Autodesk Fusion 360 part; units mm, degrees
sketch "Sketch1" plane through (0, 0, 0) normal (0, 0, 1) x (1, 0, 0)
  line L0 (30, 50) -> (30, 22)
  line L1 (30, 22) -> (150, 22)
  line L2 (150, 22) -> (30, 50)
  dimension "d1" = 28
  dimension "d2" = 120
extrude "Extrude1" add sketch "Sketch1" along normal blind 20
sketch "Sketch2" plane through (0, 22, 0) normal (0, -1, 0) x (1, 0, 0)
  line L0 (30, 0) -> (150, 0)
  line L1 (150, 0) -> (150, 20)
  line L2 (150, 20) -> (30, 20)
  line L3 (30, 20) -> (30, 0)
  line L4 (30, 10) -> (150, 10)
  line L5 (150, 10) -> (120, 10)
  circle A0 centre (120, 10) radius 2.5
  circle A1 centre (65, 10) radius 2.5
  dimension "d5" = 30
  dimension "d6" = 5
  dimension "d7" = 5
extrude "Extrude2" cut sketch "Sketch2" against normal blind 50 contours L4 A1 | L4 A1 | L4 L5 A0 | L4 L5 A0
sketch "Sketch3" plane through (0, 0, 20) normal (0, 0, 1) x (-1, 0, 0)
  line L0 (-150, -22) -> (-30, -50)
  line L1 (-30, -50) -> (-30, -22)
  line L2 (-30, -22) -> (-150, -22)
  line L3 (-30, -50) -> (-150, -50)
  line L4 (-150, -50) -> (-150, -22)
sketch "Sketch4" plane through (0, 22, 0) normal (0, -1, 0) x (1, 0, 0)
  circle A0 centre (65, 10) radius 2.5
  circle A1 centre (120, 10) radius 2.5
  line L0 (30, 0) -> (150, 0)
  line L1 (150, 0) -> (150, 20)
  line L2 (150, 20) -> (30, 20)
  line L3 (30, 20) -> (30, 0)
  line L4 (65, 10) -> (65, 20)
  line L5 (120, 10) -> (120, 20)
sketch "Sketch5" plane through (0, 0, 20) normal (0, 0, 1) x (-1, 0, 0)
  line L0 (-120, -22) -> (-120, -50)
  line L1 (-120, -50) -> (-65, -22)
  line L2 (-65, -22) -> (-65, -50)
sketch "Sketch6" plane through (90, 22, 10) normal (0, -1, 0) x (1, 0, 0)
  line L0 (30, 14.4) -> (40.6132, 4.6089)
sketch "Sketch7" plane through (0, 0, 0) normal (0, 0, -1) x (1, 0, 0)
  line L0 (30, -50) -> (150, -22)
  line L1 (150, -22) -> (30, -22)
  line L2 (30, -22) -> (30, -50)
Geometry check sheet. Reference: the model listing, model coordinates, mm. Give positions to 0.01 mm unless a question says otherwise; leave off trailing zeros. Loops run counter-clockwise (first coordinate to the right, second up) from the corner with the lowest first, then second, coordinate; pieces in that order, holes last.
(1) Section check A-A on x = 120. Record the cut outline in (y, z), then the cut area to 3 significant figures.
From the geometry:
outline: (22, 0) - (29, 0) - (29, 7.5) - (22, 7.5) - close; (22, 12.5) - (29, 12.5) - (29, 20) - (22, 20) - close
area: 105 mm2
(2) Thickness scan on L1, parallel to Z at x = 120, y = 27.25; L2, parallel to Y at x = 87, z = 10; L3, parallel to Y at x = 129, z = 16.5. Record the ranges inside material, lowest first.
From the geometry:
L1: z = 0 to 7.5, 12.5 to 20
L2: y = 22 to 36.7
L3: y = 22 to 26.9
(3) Section check C-C on z = 10. Record the cut outline in (x, y).
From the geometry:
outline: (30, 22) - (62.5, 22) - (62.5, 42.42) - (30, 50) - close; (67.5, 22) - (117.5, 22) - (117.5, 29.58) - (67.5, 41.25) - close; (122.5, 22) - (150, 22) - (122.5, 28.42) - close
(4) Section check D-D on y = 27. Record the cut outline in (x, z).
From the geometry:
outline: (30, 0) - (128.57, 0) - (128.57, 20) - (30, 20) - close; hole circle Ø5 at (65, 10); hole circle Ø5 at (120, 10)
(5) Depth check by flat-ended pin: pin 1 Ø3 at (x, z) = (61.5, 3) entering from +Y; pin 2 Ø8 at (x, z) = (65, 10) entering from +Y. Enter the tip coordinate at first touch or a pass-through.
From the geometry:
pin 1: stops at y = 43
pin 2: stops at y = 42.77
(6) Section check B-B on y = 37.75. Record the cut outline in (x, z).
From the geometry:
outline: (30, 0) - (82.5, 0) - (82.5, 20) - (30, 20) - close; hole circle Ø5 at (65, 10)
(7) Release check for a two-part mould opening along X. For faces 1 (the flat face through (90.84, 35.804, 9.86)), 2 (the flat face through (89, 22, 10)), 3 (the cylindrical face through (118, 25.7, 8.5)), 4 (the cylindrical face through (66.15, 32.07, 7.78)) record: released by +X, released by -X, zero draft, split by the parting line, or undercut.
From the geometry:
face 1: released by +X
face 2: zero draft
face 3: undercut
face 4: undercut
